Read the model definition and answer for the solid it produces. Units are mm, in the model's axes. A direction names the side the tool comes from. Coordinates: 2 decimals unless noted, no trailing zeros. Loops run counter-clockwise (first coordinate to the right, second up) from the corner with the lowest first, then second, coordinate; pieces in that order, holes last. Notation, with made-up numbers: (69, -28.5) -> (122, -28.5) arc R8 cw to (122, -23.5) -> close; hole circle Ø9 at (54, 79.5). An arc over 180 degrees is marked (long way). Answer as a JSON object with one key per item and string values. Group by question number.
1) Consider probe 1 along Z at (x, y) = (8, 2.4); probe 2 along X at (y, z) = (1.65, 8); probe 3 along Z at (x, y) = (-17, 16). Determine where each line is inside the solid, lowest interval first. Write a range as [from, to].
2) Section A-A, the plane y = 4.75 is taken. Give the vertices of the cut face in (x, z), plus the area to 3 significant figures.
3) Section D-D, the plane x = 16.5 is taken. Give the vertices of the cut face in (y, z), plus the area to 3 significant figures.
4) Section B-B, the plane z = -8 is taken. Give the vertices of the cut face in (x, y), plus the area to 3 significant figures.
5) Which of the six approach directions +Z, -Z, +X, -X, +Y, -Y give full straight-line access (tool end or side, diameter ignored) to faces 1 (the face through (-24.5, 2, 0)), 2 (the face through (15, 19, -20)), 3 (the face through (0, 13, -19))?
6) Section C-C, the plane x = -13 is taken. Give the vertices of the cut face in (y, z).
7) Flat-ended cylindrical pins translate along their axes: P1, Ø1.8, axis at x = 8, z = 8, coming from the +Y side; P2, Ø3.5, axis at x = 8, z = -8, coming from the +Y side. Find the tip coordinate at first contact, or state that the pin passes through.
8) Determine the mould class of faces 4 (the face through (11.5, 2, 0)), 5 (the face through (6, 3, 0)) for opening direction X: released by +X, released by -X, zero draft, split by the parting line, or undercut.
Autodesk Inventor part; units mm, degrees
ref_plane "YZ Plane" through (0, 0, 0) normal (1, 0, 0) x (0, 1, 0)
ref_plane "XZ Plane" through (0, 0, 0) normal (0, 1, 0) x (-1, 0, 0)
ref_plane "XY Plane" through (0, 0, 0) normal (0, 0, 1) x (1, 0, 0)
sketch "Szkic1" plane through (0, 0, 0) normal (0, 1, 0) x (-1, 0, 0)
  line L0 (27.5, 22) -> (-27.5, 22)
  line L1 (-27.5, 22) -> (-27.5, -22)
  line L2 (-27.5, -22) -> (27.5, -22)
  line L3 (27.5, -22) -> (27.5, 22)
  line L4 (27.5, 22) -> (-27.5, -22) construction
  line L5 (-27.5, 22) -> (27.5, -22) construction
  point P0 (0, 0)
  dimension "d0" = 55
  dimension "d1" = 44
extrude "Wyciągnięcie proste1" add sketch "Szkic1" along normal blind 3
sketch "Szkic2" plane through (0, 3, 0) normal (0, 1, 0) x (1, 0, 0)
  line L0 (27.5, 22) -> (-27.5, 22)
  line L1 (27.5, -22) -> (27.5, 22)
  line L2 (-27.5, 22) -> (27.5, 22)
  line L3 (27.5, 22) -> (27.5, 19)
  line L4 (27.5, 19) -> (-27.5, 19)
  line L5 (-27.5, 19) -> (-27.5, 22)
  line L6 (-27.5, 22) -> (-27.5, -22)
  line L7 (27.5, -22) -> (-27.5, -22)
  line L8 (-27.5, -22) -> (-27.5, -19)
  line L9 (-27.5, -19) -> (27.5, -19)
  line L10 (27.5, -19) -> (27.5, -22)
  point P0 (0, 0)
  dimension "d4" = 3
  dimension "d5" = 3
extrude "Wyciągnięcie proste2" add sketch "Szkic2" along normal blind 20 contours L1 L4 L5 L0 | L1 L7 L6 L9
sketch "Szkic4" plane through (0, 3, 0) normal (0, 1, 0) x (1, 0, 0)
  line L0 (-27.5, 19) -> (-27.5, -19)
  line L1 (-27.5, 0) -> (27.5, 0) construction
  line L2 (27.5, -19) -> (27.5, 19)
  line L3 (-27.5, -22) -> (27.5, -22)
  line L4 (0, -22) -> (0, 22) construction
  line L5 (27.5, 22) -> (-27.5, 22)
  point P0 (0, 0)
  point P1 (-8, -8)
  point P2 (-8, 8)
  point P3 (8, -8)
  point P4 (8, 8)
  dimension "d13" = 8
  dimension "d16" = 8
hole "Otwór1" at (-8, 3, 8) at (-8, 3, -8) at (8, 3, 8) at (8, 3, -8) direction (0, -1, 0) diameter 3 depth 8 tip angle 118
sketch "Szkic5" plane through (0, 3, 0) normal (0, 1, 0) x (1, 0, 0)
  line L0 (-24.5, -16) -> (-11.5, -16)
  line L1 (-11.5, -16) -> (-11.5, 16)
  line L2 (-11.5, 16) -> (-24.5, 16)
  line L3 (-24.5, 16) -> (-24.5, -16)
  line L4 (27.5, -19) -> (-27.5, -19)
  line L5 (27.5, 19) -> (-27.5, 19)
  line L6 (-27.5, 22) -> (-27.5, -22)
  line L7 (-27.5, -22) -> (27.5, -22)
  line L8 (0, -22) -> (0, 22) construction
  line L9 (27.5, 22) -> (-27.5, 22)
  line L10 (24.5, -16) -> (11.5, -16)
  line L11 (11.5, -16) -> (11.5, 16)
  line L12 (11.5, 16) -> (24.5, 16)
  line L13 (24.5, 16) -> (24.5, -16)
  point P0 (0, 0)
  dimension "d27" = 3
  dimension "d28" = 3
  dimension "d29" = 3
  dimension "d30" = 13
sketch "Szkic6" plane through (-27.5, 0, 22) normal (0, 0, 1) x (1, 0, 0)
  line L0 (12.5, 17.5) -> (42.5, 17.5)
  line L1 (42.5, 17.5) -> (42.5, 20.5)
  line L2 (42.5, 20.5) -> (12.5, 20.5)
  line L3 (12.5, 20.5) -> (12.5, 17.5)
  line L4 (12.5, 17.5) -> (42.5, 20.5) construction
  line L5 (42.5, 17.5) -> (12.5, 20.5) construction
  line L6 (55, 23) -> (0, 23)
  line L7 (55, 0) -> (55, 23)
  point P0 (27.5, 0)
  point P1 (27.5, 19)
  dimension "d33" = 30
  dimension "d34" = 3
  dimension "d35" = 4
  dimension "d36" = 27.5
extrude "Wyciągnięcie proste4" cut sketch "Szkic6" against normal through all
extrude "Wyciągnięcie proste5" cut sketch "Szkic5" against normal blind 10
properties part number "Li-Pol_uchwyt" material "Tworzywo sztuczne PET"
Determined:
{
 "1": {"probe 1": "[-22, -9.5], [-6.5, 6.5], [9.5, 22]", "probe 2": "[-27.5, -24.5], [-11.5, -9.5], [-6.5, 6.5], [9.5, 11.5], [24.5, 27.5]", "probe 3": "[-22, -19], [19, 22]"},
 "2": {"outline": "(-27.5, -22) -> (27.5, -22) -> (27.5, -19) -> (-27.5, -19) -> close; (-27.5, 19) -> (27.5, 19) -> (27.5, 22) -> (-27.5, 22) -> close", "area": "330 mm²"},
 "3": {"outline": "(0, -22) -> (23, -22) -> (23, -19) -> (3, -19) -> (3, -16) -> (0, -16) -> close; (0, 16) -> (3, 16) -> (3, 19) -> (23, 19) -> (23, 22) -> (0, 22) -> close", "area": "156 mm²"},
 "4": {"outline": "(-27.5, 0) -> (-24.5, 0) -> (-24.5, 3) -> (-27.5, 3) -> close; (-11.5, 0) -> (-9.5, 0) -> (-9.5, 3) -> (-11.5, 3) -> close; (-6.5, 0) -> (6.5, 0) -> (6.5, 3) -> (-6.5, 3) -> close; (9.5, 0) -> (11.5, 0) -> (11.5, 3) -> (9.5, 3) -> close; (24.5, 0) -> (27.5, 0) -> (27.5, 3) -> (24.5, 3) -> close", "area": "69.0 mm²"},
 "5": {"face 1": "+Y, -Y", "face 2": "+Z, -Z", "face 3": "+X, -X, +Y"},
 "6": {"outline": "(0, -22) -> (17.5, -22) -> (17.5, -19) -> (3, -19) -> (3, -16) -> (0, -16) -> close; (0, 16) -> (3, 16) -> (3, 19) -> (17.5, 19) -> (17.5, 22) -> (0, 22) -> close; (20.5, -22) -> (23, -22) -> (23, -19) -> (20.5, -19) -> close; (20.5, 19) -> (23, 19) -> (23, 22) -> (20.5, 22) -> close"},
 "7": {"P1": "through", "P2": "y = 3"},
 "8": {"face 4": "undercut", "face 5": "zero draft"}
}
